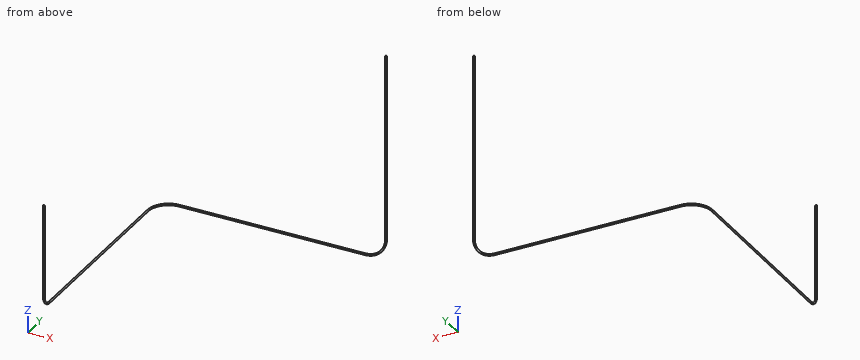
```python
from build123d import *

# Parameters (mm, degrees)
SKETCH1_R = 2


with BuildPart() as part:
    # Sweep1: sweep along a curve in space
    with BuildLine() as sweep1_path:
        Line((0, 0, 0), (0, 0, -450))
        ThreePointArc((0, 0, -450), (-14.644660941, 0, -485.355339059), (-50, 0, -500))
        Line((-50, 0, -500), (-500, 0, -500))
        ThreePointArc((-500, 0, -500), (-535.355339059, -14.644660941, -500), (-550, -50, -500))
        Line((-550, -50, -500), (-550, -500, -500))
        ThreePointArc((-550, -525, -475), (-550, -517.67766953, -492.67766953), (-550, -500, -500))
        Line((-550, -525, -475), (-550, -525, -250))
    # Sketch1 → Sweep1 (sweep)
    with BuildSketch(Plane.XY):
        Circle(SKETCH1_R)
    sweep(path=sweep1_path.line)


solid = part.part
```
CAD build for the part. Positions are in the model's coordinates, mm. Coordinates: 2 decimals unless noted, no trailing zeros. Order: outer loops, then holes, each group sorted by start corner. A loop starts at its lowest first (then second) coordinate and runs counter-clockwise, first axis right, second up. Notation, with made-up numbers: (68.25, -11.5) -> (112.25, -11.5) arc R24 ccw to (112.25, -0.5) -> close; hole circle Ø6 at (67.25, 55). An arc over 180 degrees is marked (long way). Use one line per item in the form item = value. Start each with the question number.
1) Band-saw the part on A-A on z = -432.5. Give the cut face in (x, y).
2) Drop a flat-ended pin along its axis: pin 1 (3 mm diameter, centred on x = -550, y = -525.5, fed in from +Z). Give the stop position or say it passes through.
3) Band-saw the part on B-B on x = -61. Give the cut face in (y, z), then the cut area to 3 significant figures.
4) Band-saw the part on C-C on z = -231. Give the cut face in (x, y), then the cut area to 3 significant figures.
Entries:
q1.outline = circle Ø4 at (-550, -525); circle Ø4 at (0, 0)
q2.pin_1 = -250
q3.outline = circle Ø4 at (0, -500)
q3.area = 12.6 mm2
q4.outline = circle Ø4 at (0, 0)
q4.area = 12.6 mm2
